from build123d import *

# Parameters (mm, degrees)
SKETCH1_R           = 24
SKETCH1_R_2         = 20
BOSS_EXTRUDE1_DEPTH = 18
BOSS_EXTRUDE2_START = -3
SKETCH2_R           = 24
SKETCH2_R_2         = 10.5
SKETCH2_R_3         = 1.6
BOSS_EXTRUDE2_DEPTH = 3
SKETCH3_R           = 29
SKETCH3_R_2         = 20
SKETCH3_R_3         = 1.6
BOSS_EXTRUDE3_DEPTH = 2


with BuildPart() as part:
    # Sketch1 → Boss-Extrude1 (new body)
    with BuildSketch(Plane(origin=(0, 0, 0), x_dir=(1, 0, 0), z_dir=(0, 1, 0))):
        with Locations(Location((0, 0, 0), (0, 0, 270))):
            Circle(SKETCH1_R)
        with Locations(Location((0, 0, 0), (0, 0, 270))):
            Circle(SKETCH1_R_2, mode=Mode.SUBTRACT)
    extrude(amount=BOSS_EXTRUDE1_DEPTH)

    # Sketch2 → Boss-Extrude2 (add)
    with BuildSketch(Plane(origin=(0, 0, 0), x_dir=(1, 0, 0), z_dir=(0, 1, 0)).offset(BOSS_EXTRUDE2_START)):
        with Locations(Location((0, 0, 0), (0, 0, 270))):
            Circle(SKETCH2_R)
        with Locations(Location((0, 0, 0), (0, 0, 270))):
            Circle(SKETCH2_R_2, mode=Mode.SUBTRACT)
        with Locations(Location((0, 15, 0), (0, 0, 270))):
            Circle(SKETCH2_R_3, mode=Mode.SUBTRACT)
        with Locations(Location((12.990381057, -7.5, 0), (0, 0, 270))):
            Circle(SKETCH2_R_3, mode=Mode.SUBTRACT)
        with Locations(Location((-12.990381057, -7.5, 0), (0, 0, 270))):
            Circle(SKETCH2_R_3, mode=Mode.SUBTRACT)
    extrude(amount=BOSS_EXTRUDE2_DEPTH)

    # Sketch3 → Boss-Extrude3 (add)
    with BuildSketch(Plane(origin=(0, 18, 0), x_dir=(1, 0, 0), z_dir=(0, 1, 0))):
        with Locations(Location((0, 0, 0), (0, 0, 270))):
            Circle(SKETCH3_R)
        with Locations(Location((0, 0, 0), (0, 0, 270))):
            Circle(SKETCH3_R_2, mode=Mode.SUBTRACT)
        with Locations(Location((-26.5, 0, 0), (0, 0, 270))):
            Circle(SKETCH3_R_3, mode=Mode.SUBTRACT)
        with Locations(Location((13.25, 22.9496732, 0), (0, 0, 270))):
            Circle(SKETCH3_R_3, mode=Mode.SUBTRACT)
        with Locations(Location((13.25, -22.9496732, 0), (0, 0, 270))):
            Circle(SKETCH3_R_3, mode=Mode.SUBTRACT)
    extrude(amount=BOSS_EXTRUDE3_DEPTH)


solid = part.part
Geometry: final body of the model. Coordinates: model frame, mm. A direction names the side the tool comes from. Round coordinates to 2 decimals unless told otherwise and drop trailing zeros. Write each loop counter-clockwise with the first axis right and the second up, starting at its lowest first coordinate (ties: lowest second). Pieces come first, ordered by that corner, then holes. Notation, with made-up numbers: M 78,40 L 106,40 A7 ccw 106,51 Z; hole C 71.25,67.25 d1. An arc over 180 degrees is marked long. Write item = value, one per line.
Item 1: Access query for faces 1 (the face through (14.836, 18.986, -23.158)), 2 (the face through (-19.524, 9.86, -4.336)), 3 (the face through (22, 18, -11)). Directions: +Z, -Z, +X, -X, +Y, -Y. A direction counts if a zero-diameter tool reaches every point of the face in a straight line with its end or side. Return the directions, or none.
Findings:
face_1 = +Y, -Y
face_2 = +Y
face_3 = -Y
Item 2: Material intervals for line 1 along X through (y, z) = (-1.5, 7.5); line 2 along Y through (x, z) = (2, 15.5); line 3 along X through (y, z) = (11, 17), sorted ascending. Write a range as [from, to].
Findings:
line_1 = [-22.8, -14.59], [-11.39, -7.35], [7.35, 11.39], [14.59, 22.8]
line_2 = [-3, 0]
line_3 = [-16.94, -10.54], [10.54, 16.94]
Item 3: Section query A-A on x = 0. Return loops of the section in (y, z).
Findings:
outline = M -3,-24 L 18,-24 L 18,-29 L 20,-29 L 20,-20 L 0,-20 L 0,-16.6 L -3,-16.6 Z; M -3,-13.4 L 0,-13.4 L 0,-10.5 L -3,-10.5 Z; M -3,10.5 L 0,10.5 L 0,20 L 20,20 L 20,29 L 18,29 L 18,24 L -3,24 Z
Item 4: Section query B-B on z = 7.5. Return loops of the section in (x, y), then the cut area to 3 significant figures.
Findings:
outline = M -28.01,18 L -22.8,18 L -22.8,-3 L -14.59,-3 L -14.59,0 L -18.54,0 L -18.54,20 L -28.01,20 Z; M -11.39,-3 L -7.35,-3 L -7.35,0 L -11.39,0 Z; M 7.35,-3 L 11.39,-3 L 11.39,0 L 7.35,0 Z; M 14.59,-3 L 22.8,-3 L 22.8,18 L 28.01,18 L 28.01,20 L 18.54,20 L 18.54,0 L 14.59,0 Z
area = 265 mm^2
Item 5: Pull-direction query (Z, two-part tool) for faces 4 (the face through (-5, -3, 10)), 5 (the face through (7.21, 7.35, 22.89)), 6 (the face through (-9, 0, 9)); classes: pulls with the +Z half, pulls with the -Z half, needs draft (parallel to the pull), parting line crosses it, or undercut.
Findings:
face_4 = needs draft
face_5 = parting line crosses it
face_6 = undercut
Item 6: Section query C-C on x = 7. Return loops of the section in (y, z) (1 decimal), then the cut area to 3 significant figures.
Findings:
outline = M -3,-23 L 18,-23 L 18,-28.1 L 20,-28.1 L 20,-18.7 L 0,-18.7 L 0,-7.8 L -3,-7.8 Z; M -3,7.8 L 0,7.8 L 0,18.7 L 20,18.7 L 20,28.1 L 18,28.1 L 18,23 L -3,23 Z
area = 280 mm^2
Item 7: Section query D-D on z = -15. Return loops of the section in (x, y) (3 decimals), then the cut area to 3 significant figures.
Findings:
outline = M -24.819,18 L -18.735,18 L -18.735,-3 L -1.6,-3 L -1.6,0 L -13.229,0 L -13.229,20 L -24.819,20 Z; M 1.6,-3 L 18.735,-3 L 18.735,18 L 24.819,18 L 24.819,20 L 13.229,20 L 13.229,0 L 1.6,0 Z
area = 347 mm^2
Item 8: Pin query (flat end, axial travel): P1, Ø10, axis at x = 18, y = 8, coming from the +Z side; P2, Ø3, axis at x = 13, y = -0.5, coming from the +Z side; P3, Ø12, axis at x = 3, z = 4, coming from the +Y side. Return the tip coordinate at first contact, or that it passes through.
Findings:
P1 = 20.17
P2 = 21.07
P3 = 0
